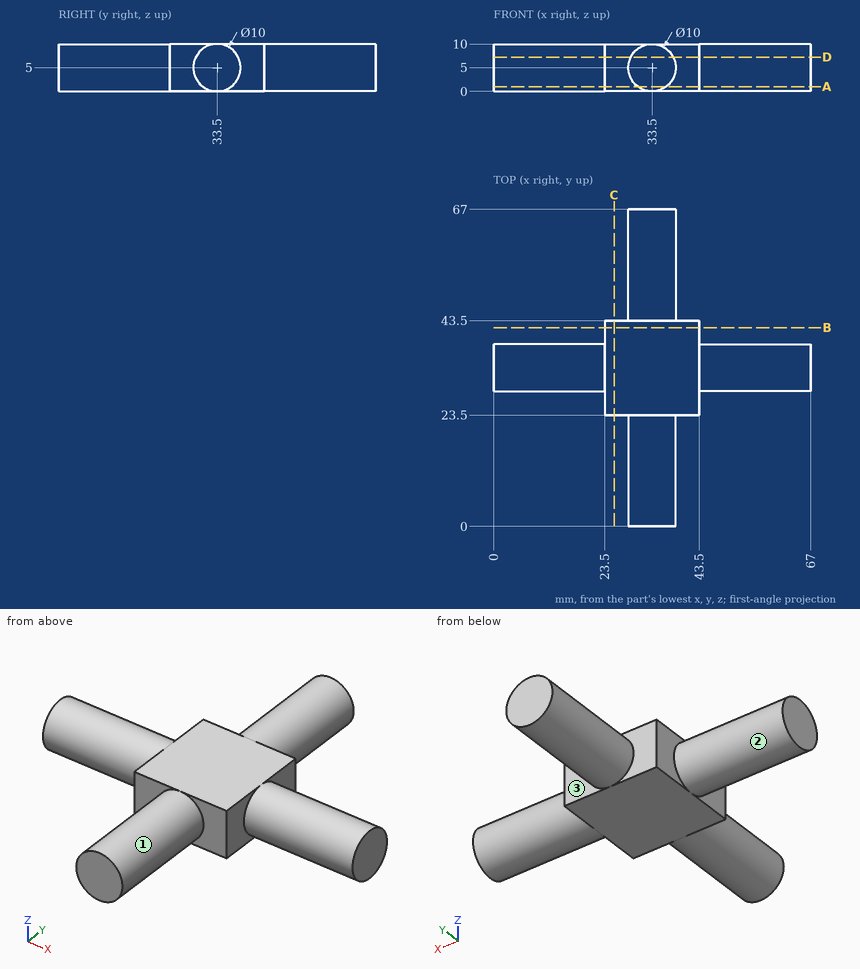
The drawing under review shows one solid part. Ordinate dimensions are in mm from its lowest x, y, z. A direction names the side the tool comes from. Give positions to 0.01 mm unless a question says otherwise; leave off trailing zeros. Loops run counter-clockwise (first coordinate to the right, second up) from the corner with the lowest first, then second, coordinate; pieces in that order, holes last. Notation, with made-up numbers: M 70.5,-6.75 L 128.5,-6.75 A23 cw 128.5,16.25 Z; hole C 29.5,86 d4. An arc over 180 degrees is marked long. Return JSON: item names as keys, results as strings. Group by question number.
Item 1: Tool access review of the marked faces 1, 2 and 3: name each direction out of +Z, -Z, +X, -X, +Y, -Y from which nothing blocks a thin tool from reaching the whole face with its end or side.
Item 2: For probe 1 along Y at (x, z) = (26, 7.5); probe 2 along X at (y, z) = (22, 2), list the stretches that pass through material, from the lowest coordinate up.
Item 3: Insertion check: pin 1 Ø1 at (x, y) = (8.5, 37) entering from +Z; pin 2 Ø6 at (x, z) = (8, 2) entering from -Y; pin 3 Ø12 at (x, y) = (25.5, 57) entering from +Z. Each pin has a flat end and moves straight along its axis. Give the tip position at first contact, or say it passes through.
Item 4: We need section D-D (z = 7.25). Give the boundary of the cut face in (x, y), and give its area (3 significant figures).
Item 5: We need section A-A (z = 1). Give the boundary of the cut face in (x, y).
Item 6: We need section B-B (y = 42). Give the boundary of the cut face in (x, z).
Output:
{
 "1": {"face 1": "-Y", "face 2": "-X", "face 3": "+X, +Y"},
 "2": {"probe 1": "y = 23.5 to 43.5", "probe 2": "x = 29.5 to 37.5"},
 "3": {"pin 1": "stops at z = 9", "pin 2": "stops at y = 28.5", "pin 3": "stops at z = 9.58"},
 "4": {"outline": "M 0,29.03 L 23.5,29.03 L 23.5,23.5 L 29.03,23.5 L 29.03,0 L 37.97,0 L 37.97,23.5 L 43.5,23.5 L 43.5,29.03 L 67,29.03 L 67,37.97 L 43.5,37.97 L 43.5,43.5 L 37.97,43.5 L 37.97,67 L 29.03,67 L 29.03,43.5 L 23.5,43.5 L 23.5,37.97 L 0,37.97 Z", "area": "1,240 mm^2"},
 "5": {"outline": "M 0,30.5 L 23.5,30.5 L 23.5,23.5 L 30.5,23.5 L 30.5,0 L 36.5,0 L 36.5,23.5 L 43.5,23.5 L 43.5,30.5 L 67,30.5 L 67,36.5 L 43.5,36.5 L 43.5,43.5 L 36.5,43.5 L 36.5,67 L 30.5,67 L 30.5,43.5 L 23.5,43.5 L 23.5,36.5 L 0,36.5 Z"},
 "6": {"outline": "M 23.5,0 L 43.5,0 L 43.5,10 L 23.5,10 Z"}
}
